Job drawing, mm, ordinate dimensions from the low corner. One solid piece. A direction names the side the tool comes from. Round coordinates to 2 decimals unless told otherwise and drop trailing zeros. Loops run counter-clockwise (first coordinate to the right, second up) from the corner with the lowest first, then second, coordinate; pieces in that order, holes last.
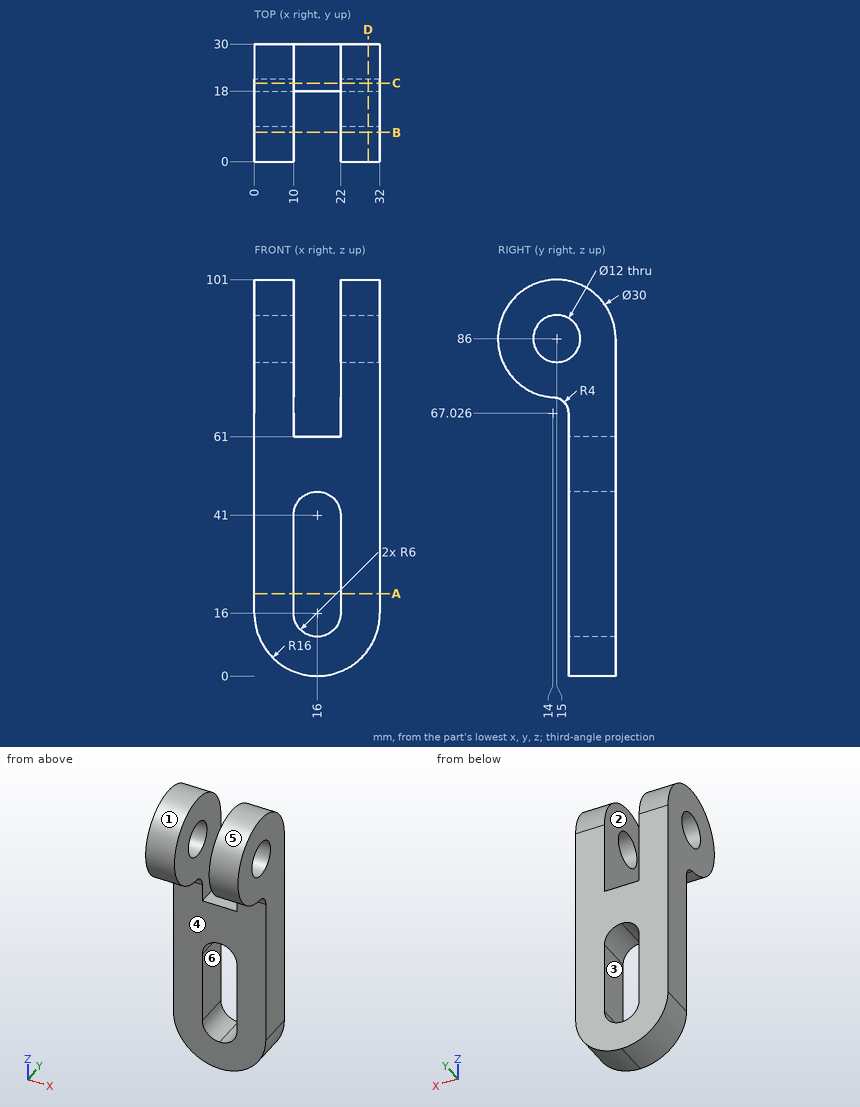
Item 1: Cut at B-B, the plane y = 7.5. Give the cut face in (x, z).
Answers follow:
outline: (0, 73.01) - (10, 73.01) - (10, 98.99) - (0, 98.99) - close; (22, 73.01) - (32, 73.01) - (32, 98.99) - (22, 98.99) - close
Item 2: Probe line 1 (X direction, y = 19.5, z = 41); line 2 (Y direction, x = 5.5, z = 62.5); line 3 (Z direction, x = 13, y = 21.5) (1 decimal). List the from-to ranges inside material, lowest first.
Answers follow:
line 1: x = 0 to 10, 22 to 32
line 2: y = 18 to 30
line 3: z = 0.3 to 10.8, 46.2 to 61
Item 3: Flat gauge pins, fed straight in: P1, Ø1, axis at x = 6, y = 16, coming from the -Z side; P2, Ø6, axis at x = 9, y = 23.5, coming from the -Z side; P3, Ø6, axis at x = 16.5, y = 24, coming from the +Z side. Where does each tip first touch, or does it go through?
Answers follow:
P1: stops at z = 70.15
P2: stops at z = 0.51
P3: stops at z = 61
Item 4: 3-axis set-ups, long thin cutter, end or side, ignore diameter. For the marked faces 1 and 2: which of +Z, -Z, +X, -X, +Y, -Y reach the whole face in a straight line?
Answers follow:
face 1: +X, -X
face 2: +Z, +Y, -Y
Item 5: Two-plate mould, pull along Z, no slides. Class the marked faces 3, 4, 5 and 6: released by +Z, released by -Z, zero draft, split by the parting line, or undercut.
Answers follow:
face 3: undercut
face 4: zero draft
face 5: split by the parting line
face 6: undercut
Item 6: Cut at A-A, the plane z = 21. Give the cut face in (x, y).
Answers follow:
outline: (0, 18) - (10, 18) - (10, 30) - (0, 30) - close; (22, 18) - (32, 18) - (32, 30) - (22, 30) - close
Item 7: Cut at D-D, the plane x = 29. Give the cut face in (y, z), plus the area to 3 significant figures.
Answers follow:
outline: (14.21, 71.02) arc R4 cw to (18, 67.03) - (18, 6.67) - (30, 6.67) - (30, 86) arc R15 ccw (long way) to start; hole circle Ø12 at (15, 86)
area: 1,420 mm2
Item 8: Cut at C-C, the plane y = 20. Give the cut face in (x, z).
Answers follow:
outline: (0, 16) arc R16 ccw to (16, 0) arc R16 ccw to (32, 16) - (32, 82.68) - (22, 82.68) - (22, 61) - (10, 61) - (10, 82.68) - (0, 82.68) - close; (0, 89.32) - (10, 89.32) - (10, 100.14) - (0, 100.14) - close; (22, 89.32) - (32, 89.32) - (32, 100.14) - (22, 100.14) - close; hole (10, 16) arc R6 ccw to (16, 10) arc R6 ccw to (22, 16) - (22, 41) arc R6 ccw to (16, 47) arc R6 ccw to (10, 41) - close
